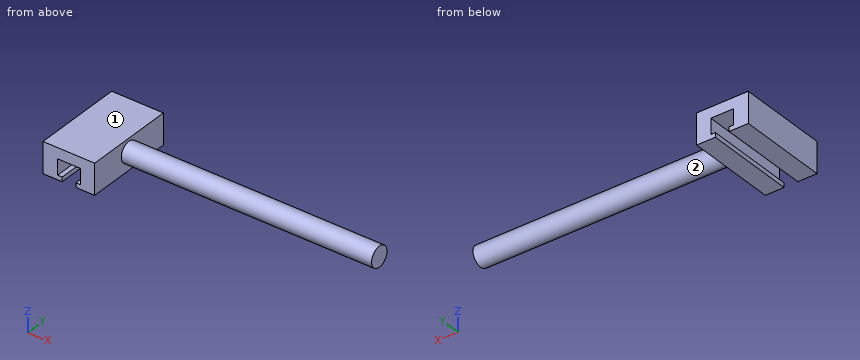
from build123d import *

# Parameters (mm, degrees)
F1_DEPTH = 25.4
F2_DEPTH = 4.572
F3_R     = 2.8483502815
F4_DEPTH = 70.104
F5_DEPTH = 1.27
F6_W     = 25.4
F6_H     = 1.2553478565
F8_DEPTH = 1.27
F7_W     = 25.4
F7_H     = 1.2564980398
F9_DEPTH = 1.27


with BuildPart() as f1:
    # F0 (on Front) → F1 (new body)
    with BuildSketch(Plane.XZ):
        Polygon((0, 11.9274239987), (0, 0), (4.1132315528, 0), (4.1132315528, 8.9138071053), (10.4970876127, 8.9138071053), (10.4970876127, 0), (14.4736012444, 0), (14.4736012444, 11.9274239987), align=None)
    extrude(amount=F1_DEPTH)

    # F2 (cut): faces of the model
    f2_faces = [f1.faces().sort_by_distance(p)[0] for p in [
        (2.0566157764, -12.7, 0),
        (12.4853444286, -12.7, 0),
    ]]
    extrude(f2_faces, amount=-F2_DEPTH, mode=Mode.SUBTRACT)

    # F3 (on face) → F4 (join)
    with BuildSketch(Plane.YZ.offset(14.4736012444)):
        with Locations((-12.7, 8.2497119994)):
            Circle(F3_R)
    extrude(amount=F4_DEPTH)

    # F5 (add): faces of the model
    f5_faces = [f1.faces().sort_by_distance(p)[0] for p in [
        (12.4853444286, -12.7, 4.572),
        (2.0566157764, -12.7, 4.572),
    ]]
    extrude(f5_faces, amount=F5_DEPTH)

    # F6 (on face) → F8 (join)
    with BuildSketch(Plane(origin=(10.4970876127, 0, 0), x_dir=(0, -1, 0), z_dir=(-1, 0, 0))):
        with Locations((12.7, 3.9296739282)):
            Rectangle(F6_W, F6_H)
    extrude(amount=F8_DEPTH)

    # F7 (on face) → F9 (join)
    with BuildSketch(Plane.YZ.offset(4.1132315528)):
        with Locations((-12.7, 3.9302490199)):
            Rectangle(F7_W, F7_H)
    extrude(amount=F9_DEPTH)


solid = f1.part
Build history of the part. All positions in model axes, mm. Face numbers are marked on the shaded views. A direction names the side the tool comes from. Give positions to 0.01 mm unless a question says otherwise; leave off trailing zeros. Write each loop counter-clockwise with the first axis right and the second up, starting at its lowest first coordinate (ties: lowest second). Pieces come first, ordered by that corner, then holes. Notation, with made-up numbers: (-30, 44.5) - (10, 44.5) arc R13 ccw to (10, 50.5) - close; hole circle Ø7 at (-5.5, -32.75). An arc over 180 degrees is marked (long way). Use one line per item in the form item = value. Start each with the question number.
1. Probe line 1 (X direction, y = -12.25, z = 7.5); line 2 (X direction, y = -16, z = 5.25); line 3 (X direction, y = -17, z = 9). List the from-to ranges inside material, lowest first. Write a range as [from, to].
2. Drop flat-ended pins along their axis: pin 1 Ø1.5 at (x, z) = (26.5, 11) entering from +Y; pin 2 Ø6 at (x, y) = (43, -19) entering from -Z. Give the stop position or say it passes through.
3. 3-axis set-ups, long thin cutter, end or side, ignore diameter. For the marked faces 1 and 2: which of +Z, -Z, +X, -X, +Y, -Y reach the whole face in a straight line?
4. Band-saw the part on D-D on x = 44.5. Write the cut outline in (y, z).
5. Band-saw the part on B-B on z = 7.25. Write the cut outline in (x, y).
6. Band-saw the part on A-A on y = -9. Write the cut outline in (x, z), plus the area to 3 significant figures.
7. Band-saw the part on C-C on y = -12.7. Write the cut outline in (x, z), plus the area to 3 significant figures.
Conclusion:
q1.line_1 = [0, 4.11], [10.5, 84.58]
q1.line_2 = [0, 4.11], [10.5, 14.47]
q1.line_3 = [0, 14.47]
q2.pin_1 = -10.67
q2.pin_2 = through
q3.face_1 = +Z, +X, -X, +Y, -Y
q3.face_2 = +X
q4.outline = circle Ø5.7 at (-12.7, 8.25)
q5.outline = (0, -25.4) - (4.11, -25.4) - (4.11, 0) - (0, 0) - close; (10.5, -25.4) - (14.47, -25.4) - (14.47, -15.37) - (84.58, -15.37) - (84.58, -10.03) - (14.47, -10.03) - (14.47, 0) - (10.5, 0) - close
q6.outline = (0, 3.3) - (5.38, 3.3) - (5.38, 4.56) - (4.11, 4.56) - (4.11, 8.91) - (10.5, 8.91) - (10.5, 4.56) - (9.23, 4.56) - (9.23, 3.3) - (14.47, 3.3) - (14.47, 11.93) - (0, 11.93) - close
q6.area = 92.2 mm²
q7.outline = (0, 3.3) - (5.38, 3.3) - (5.38, 4.56) - (4.11, 4.56) - (4.11, 8.91) - (10.5, 8.91) - (10.5, 4.56) - (9.23, 4.56) - (9.23, 3.3) - (14.47, 3.3) - (14.47, 5.4) - (84.58, 5.4) - (84.58, 11.1) - (14.47, 11.1) - (14.47, 11.93) - (0, 11.93) - close
q7.area = 492 mm²
